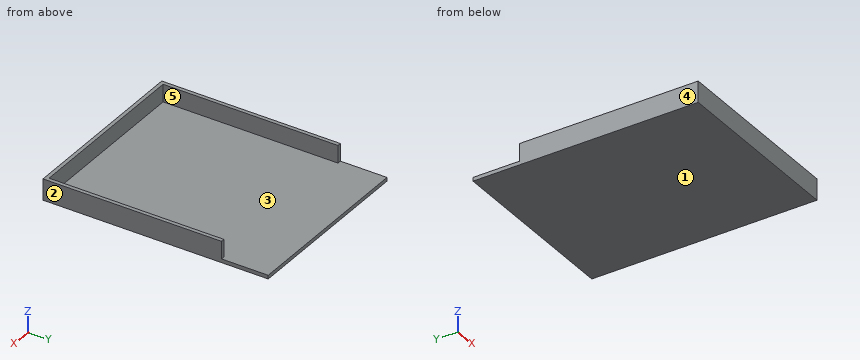
Autodesk Inventor part; units mm, degrees
ref_plane "YZ Plane" through (0, 0, 0) normal (1, 0, 0) x (0, 1, 0)
ref_plane "XZ Plane" through (0, 0, 0) normal (0, 1, 0) x (-1, 0, 0)
ref_plane "XY Plane" through (0, 0, 0) normal (0, 0, 1) x (1, 0, 0)
sketch "Sketch1" plane through (0, 0, 0) normal (0, 1, 0) x (-1, 0, 0)
  line L0 (0, 0) -> (95.25, 0)
  line L1 (95.25, 0) -> (95.25, -9.525)
  line L2 (95.25, -9.525) -> (0, -9.525)
  line L3 (0, -9.525) -> (0, 0)
  line L4 (-2, -11.525) -> (97.25, -11.525)
  line L5 (97.25, -11.525) -> (97.25, 2)
  line L6 (97.25, 2) -> (-2, 2)
  line L7 (-2, 2) -> (-2, -11.525)
  line L8 (95.25, 0) -> (97.25, 0)
  line L9 (0, 0) -> (-2, 0)
  dimension "d0" = 95.25
  dimension "d1" = 9.525
  dimension "d4" = 2
extrude "Extrusion1" add sketch "Sketch1" along normal blind 2 contours L0 L1 L2 L3 | L3 L2 L1 L8 L5 L4 L7 L9
sketch "Sketch2" plane through (0, 2, 0) normal (0, 1, 0) x (1, 0, 0)
  line L0 (-97.25, 0) -> (2, 0)
  line L1 (2, 0) -> (2, 11.525)
  line L2 (2, 11.525) -> (-97.25, 11.525)
  line L3 (-97.25, 11.525) -> (-97.25, 0)
  line L4 (0, 9.525) -> (0, 2)
  line L5 (0, 2) -> (-95.25, 2)
  line L6 (-95.25, 2) -> (-95.25, 9.525)
  line L7 (-95.25, 9.525) -> (0, 9.525)
  line L8 (0, 2) -> (0, 0)
  line L9 (-95.25, 2) -> (-95.25, 0)
  dimension "d5" = 2
extrude "Extrusion2" add sketch "Sketch2" along normal blind 95.25 contours L3 L2 L1 L0 L8 L4 L7 L6 L9
sketch "Sketch3" plane through (0, 97.25, 0) normal (0, 1, 0) x (1, 0, 0)
  line L0 (-97.25, 0) -> (-95.25, 0)
  line L1 (-95.25, 0) -> (-95.25, 9.525)
  line L2 (-95.25, 9.525) -> (0, 9.525)
  line L3 (0, 9.525) -> (0, 0)
  line L4 (0, 0) -> (2, 0)
  line L5 (2, 0) -> (2, 11.525)
  line L6 (2, 11.525) -> (-97.25, 11.525)
  line L7 (-97.25, 11.525) -> (-97.25, 0)
  line L8 (-97.25, 11.525) -> (2, 11.525)
  line L9 (2, 11.525) -> (2, 9.525)
  line L10 (2, 9.525) -> (-97.25, 9.525)
  line L11 (-97.25, 9.525) -> (-97.25, 11.525)
  dimension "d8" = 99.25
extrude "Extrusion3" add sketch "Sketch3" along normal blind 25.4 contours L7 L6 L5 L10 L2
properties part number "back"
The model under review builds one solid part; all positions refer to its coordinate system, in mm. Face numbers are marked on the shaded views. A direction names the side the tool comes from. Round coordinates to 2 decimals unless told otherwise and drop trailing zeros. Loops run counter-clockwise (first coordinate to the right, second up) from the corner with the lowest first, then second, coordinate; pieces in that order, holes last. Notation, with made-up numbers: (-2.75, 45) -> (17.25, 45) arc R20 ccw to (17.25, 71) -> close; hole circle Ø2 at (85.25, -3). An arc over 180 degrees is marked (long way). Answer as a JSON object with one key per item and string values. Group by question number.
1) For pin 1 Ø1.6 at (x, z) = (-96.5, -5) entering from +Y; pin 2 Ø3 at (y, z) = (98, -5) entering from -X; pin 3 Ø8 at (x, y) = (-55, 104.5) entering from +Z (3 decimals), all flat-tipped, find the tip position at first contact; note any pin that passes through.
2) We need section A-A on y = 45.5. Write out the cut boundary in (x, z) (3 decimals).
3) We need section C-C on x = -17. Write out the cut boundary in (y, z) (3 decimals).
4) For the marked faces 4 and 5, list the 3-axis set-ups (+Z, -Z, +X, -X, +Y, -Y) from which the entire face can be reached by the end or side of a thin tool; tool diameter is ignored.
5) We need section D-D on y = 111. Write out the cut boundary in (x, z) (3 decimals).
6) For line 1 (X direction, y = 15, z = -4); line 2 (Z direction, x = -44, y = 51.5) (3 decimals); line 3 (Y direction, x = -32, z = -3.5), list the stretches that pass through material, from the lowest coordinate up. Write a range as [from, to].
7) Mouldability with a two-part tool opening along X and no side actions: class the marked faces 1, 2 and 3 as released by +X, released by -X, zero draft, split by the parting line, or undercut.
8) We need section B-B on z = -2. Write out the cut boundary in (x, y).
Result set:
{
 "1": {"pin 1": "y = 97.25", "pin 2": "x = -97.25", "pin 3": "z = -9.525"},
 "2": {"outline": "(-97.25, -11.525) -> (2, -11.525) -> (2, 0) -> (0, 0) -> (0, -9.525) -> (-95.25, -9.525) -> (-95.25, 0) -> (-97.25, 0) -> close"},
 "3": {"outline": "(0, -11.525) -> (122.65, -11.525) -> (122.65, -9.525) -> (2, -9.525) -> (2, 0) -> (0, 0) -> close"},
 "4": {"face 4": "+Z, -Z, -X, +Y, -Y", "face 5": "+Z, +Y"},
 "5": {"outline": "(-97.25, -11.525) -> (2, -11.525) -> (2, -9.525) -> (-97.25, -9.525) -> close"},
 "6": {"line 1": "[-97.25, -95.25], [0, 2]", "line 2": "[-11.525, -9.525]", "line 3": "[0, 2]"},
 "7": {"face 1": "zero draft", "face 2": "released by +X", "face 3": "undercut"},
 "8": {"outline": "(-97.25, 0) -> (2, 0) -> (2, 97.25) -> (0, 97.25) -> (0, 2) -> (-95.25, 2) -> (-95.25, 97.25) -> (-97.25, 97.25) -> close"}
}
